The model under review builds one solid part; all positions refer to its coordinate system, in mm. A direction names the side the tool comes from. Give positions to 0.01 mm unless a question says otherwise; leave off trailing zeros. Loops run counter-clockwise (first coordinate to the right, second up) from the corner with the lowest first, then second, coordinate; pieces in that order, holes last. Notation, with made-up numbers: (24.25, -23) - (28.25, -23) arc R15 ccw to (28.25, -8) - close; hole circle Ø2 at (-39, 20). An arc over 180 degrees is marked (long way). Answer as a JSON object with one key per item and string values.
Autodesk Inventor part; units mm, degrees
ref_plane "YZ Plane" through (0, 0, 0) normal (1, 0, 0) x (0, 1, 0)
ref_plane "XZ Plane" through (0, 0, 0) normal (0, 1, 0) x (-1, 0, 0)
ref_plane "XY Plane" through (0, 0, 0) normal (0, 0, 1) x (1, 0, 0)
sketch "Sketch1" plane through (0, 0, 0) normal (0, 0, 1) x (1, 0, 0)
  line L0 (-750, 51.5223) -> (750, 51.5223)
  line L1 (750, 51.5223) -> (750, 0)
  line L2 (750, 0) -> (-750, 0)
  line L3 (-750, 0) -> (-750, 51.5223)
  point P0 (0, 0)
  point P1 (0, 0)
  dimension "d0" = 1500
  dimension "d1" = 51.5224
extrude "Plate1" add sketch "Sketch1" along normal blind 2
sketch "Sketch2" plane through (750, 2, 0) normal (0, -1, 0) x (1, 0, 0)
  line L0 (-1500, 0) -> (0, 0)
  line L1 (0, 0) -> (0, 30)
  line L2 (0, 30) -> (-1500, 30)
  line L3 (-1500, 30) -> (-1500, 0)
edge flange "Flange1" height 30 angle 90 thickness 2 bend radius 2.75 thickness toward (0, -1, 0) relief round relief width 2 relief depth 1 edges at (0, 0, 2) wall of the first edge with corners at (-750, 2, 0) (750, 2, 0) (750, 2, 30) (-750, 2, 30)
bend "Bend1"
corner "Corner1"
sketch "Sketch5" plane through (0, 0, 0) normal (0, 0, -1) x (-1, 0, 0)
  line L0 (750, 51.5223) -> (-750, 51.5223)
  line L1 (-1, 30) -> (-1, 51.5223)
  line L2 (750, 0) -> (-750, 0)
  line L3 (-1, 30) -> (1, 30)
  line L4 (1, 30) -> (1, 51.5223)
  point P0 (0, 0)
  point P1 (0, 30)
  point P2 (0, 0)
  dimension "d27" = 2
  dimension "d28" = 30
extrude "Extrusion1" cut sketch "Sketch5" against normal through all
pattern_linear "Rectangular Pattern1" count 3 spacing 500 along (1, 0, 0) of "Extrusion1" first direction both ways yes
sketch "Sketch6" plane through (0, 0, 0) normal (0, 0, -1) x (-1, 0, 0)
  line L0 (-750, 51.5223) -> (-750, 4.75)
  circle A0 centre (-750, 51.5223) radius 22.5
  line L1 (-750, 51.5223) -> (750, 51.5223)
  line L2 (-1, 30) -> (-1, 51.5223) construction
  line L3 (-499, 51.5223) -> (-499, 30) construction
  line L4 (-499, 30) -> (-1, 30) construction
  circle A1 centre (-250, 51.5223) radius 22.5
  point P0 (0, 0)
  point P1 (-727.5, 51.5223)
  point P2 (-750, 29.0223)
  point P3 (-250, 30)
  point P4 (-227.5, 51.5223)
  point P5 (-272.5, 51.5223)
  dimension "d24" = 45
extrude "Extrusion2" cut sketch "Sketch6" against normal through all contours L1 A0 L0 | L1 A1 picked at (-748.3311, 36.7103) picked at (-248.2369, 40.5916)
mirror "Mirror1" about plane through (0, 0, 0) normal (1, 0, 0) of "Extrusion2"
sketch "Sketch7" plane through (0, 0, 2) normal (0, 0, 1) x (1, 0, 0)
  arc A0 (-750, 29.0223) -> (-727.5, 51.5223) centre (-750, 51.5223) ccw
  line L0 (-750, 4.75) -> (-750, 29.0223)
  line L1 (-750, 4.75) -> (750, 4.75)
  line L2 (750, 29.0223) -> (750, 4.75)
  arc A1 (727.5, 51.5223) -> (750, 29.0223) centre (750, 51.5223) ccw
  line L3 (501, 51.5223) -> (727.5, 51.5223)
  line L4 (501, 51.5223) -> (501, 30)
  line L5 (501, 30) -> (499, 30)
  line L6 (499, 30) -> (499, 51.5223)
  line L7 (1, 51.5223) -> (227.5, 51.5223)
  line L8 (1, 51.5223) -> (1, 30)
  line L9 (1, 30) -> (-1, 30)
  line L10 (-1, 30) -> (-1, 51.5223)
  line L11 (-499, 51.5223) -> (-272.5, 51.5223)
  line L12 (-499, 51.5223) -> (-499, 30)
  line L13 (-499, 30) -> (-501, 30)
  line L14 (-501, 30) -> (-501, 51.5223)
  line L15 (-727.5, 51.5223) -> (-501, 51.5223)
  line L16 (650, 4.75) -> (650, 51.5223) construction
  line L17 (-750, 4.75) -> (750, 4.75)
  line L18 (646, 24.6721) -> (650, 31.6003)
  line L19 (650, 31.6003) -> (654, 24.6721)
  line L20 (654, 24.6721) -> (646, 24.6721)
  line L21 (650, 31.6003) -> (650, 24.6721) construction
  line L22 (272.5, 51.5223) -> (499, 51.5223)
  arc A2 (227.5, 51.5223) -> (272.5, 51.5223) centre (250, 51.5223) ccw
  line L23 (-227.5, 51.5223) -> (-1, 51.5223)
  arc A3 (-272.5, 51.5223) -> (-227.5, 51.5223) centre (-250, 51.5223) ccw
  point P0 (0, 0)
  point P1 (650, 28.1362)
  dimension "d29" = 100
  dimension "d30" = 8
extrude "Extrusion3" [suppressed]
mirror "Mirror2" [suppressed]
sketch "Sketch8" plane through (0, 0, 2) normal (0, 0, 1) x (1, 0, 0)
  line L0 (494, 46.5223) -> (494, 34.5223) construction
  line L1 (494, 34.5223) -> (294, 34.5223) construction
  line L2 (294, 34.5223) -> (294, 46.5223) construction
  line L3 (294, 46.5223) -> (494, 46.5223) construction
  line L4 (501, 51.5223) -> (727.5, 51.5223)
  line L5 (272.5, 51.5223) -> (499, 51.5223)
  point P0 (0, 0)
  dimension "d35" = 200
  dimension "d36" = 12
  dimension "d39" = 5
  dimension "d40" = 5
mark "Mark1"
equation "\"d1\" = Стрингер_5"
equation "\"d27\" = d18"
equation "\"d2\" = Thickness"
equation "\"d3\" = BendReliefWidth"
equation "\"d4\" = BendReliefDepth"
equation "\"d5\" = MinimumRemnant"
equation "\"d6\" = TransitionRadius"
equation "\"d9\" = BendRadius"
equation "\"d10\" = CornerReliefSize"
equation "\"d11\" = GapSize"
equation "\"d12\" = JacobiRadiusSize"
equation "\"BendReliefWidth\" = Thickness"
equation "\"BendReliefDepth\" = 0.5 * Thickness"
equation "\"CornerReliefSize\" = 4 * Thickness"
equation "\"MinimumRemnant\" = 2 * Thickness"
equation "\"TransitionRadius\" = BendRadius"
equation "\"JacobiRadiusSize\" = BendRadius"
equation "\"GapSize\" = Thickness"
equation "\"d18\" = Thickness"
properties part number "МОО 065 стрингер борт ###" material "Stainless Steel"
Q1. Consider section A-A, the plane y = 39. State the section outline as (x, z) points, plus the area to 3 significant figures.
Results:
{"outline": "(-731.31, 0) - (-501, 0) - (-501, 2) - (-731.31, 2) - close; (-499, 0) - (-268.69, 0) - (-268.69, 2) - (-499, 2) - close; (-231.31, 0) - (-1, 0) - (-1, 2) - (-231.31, 2) - close; (1, 0) - (231.31, 0) - (231.31, 2) - (1, 2) - close; (268.69, 0) - (499, 0) - (499, 2) - (268.69, 2) - close; (501, 0) - (731.31, 0) - (731.31, 2) - (501, 2) - close", "area": "2,760 mm^2"}
Q2. To check wall thickness, follow probe 1 along Z at (x, y) = (-191, 19); probe 2 along Y at (x, z) = (-583, 3.5). State the ranges of each line that lie inside material, in increasing order. Write a range as [from, to].
Results:
{"probe 1": "z = [0, 2]", "probe 2": "y = [0.17, 2.3]"}
Q3. Clearance check with flat-ended pins moving along their axes: pin 1 Ø1 at (y, z) = (36, 1) entering from +X; pin 2 Ø1 at (x, z) = (181, 16.5) entering from +Y; pin 3 Ø0.6 at (y, z) = (43.5, 1.5) entering from -X. State where each tip first meets the part, or that it passes through.
Results:
{"pin 1": "stops at x = 734.2", "pin 2": "stops at y = 2", "pin 3": "stops at x = -729.1"}
Q4. Consider section B-B, the plane x = -475. State the section outline as (y, z) points.
Results:
{"outline": "(0, 4.75) arc R4.75 ccw to (4.75, 0) - (51.52, 0) - (51.52, 2) - (4.75, 2) arc R2.75 cw to (2, 4.75) - (2, 30) - (0, 30) - close"}
Q5. Consider section C-C, the plane z = 13. State the section outline as (x, y) points, plus the area to 3 significant figures.
Results:
{"outline": "(-750, 0) - (750, 0) - (750, 2) - (-750, 2) - close", "area": "3,000 mm^2"}
Q6. Consider section D-D, the plane x = -250. State the section outline as (y, z) points.
Results:
{"outline": "(0, 4.75) arc R4.75 ccw to (4.75, 0) - (29.02, 0) - (29.02, 2) - (4.75, 2) arc R2.75 cw to (2, 4.75) - (2, 30) - (0, 30) - close"}
Q7. For faces 1 (the face through (10, 2, 17)), 2 (the face through (-750, 1.5, 8.4)), list the 3-axis set-ups (+Z, -Z, +X, -X, +Y, -Y) from which the entire face can be reached by the end or side of a thin tool; tool diameter is ignored.
Results:
{"face 1": "+Z, +X, -X, +Y", "face 2": "+Z, -Z, -X, +Y, -Y"}
